from build123d import *

# Parameters (mm, degrees)
BOSS_EXTRUDE1_DEPTH = 6


with BuildPart() as part:
    # Sketch1 → Boss-Extrude1 (new body)
    with BuildSketch(Plane(origin=(0, 0, 0), x_dir=(1, 0, 0), z_dir=(0, 1, 0))):
        with BuildLine():
            ThreePointArc((-521.750777563, 295.459449184), (-519.268832109, 299.8), (-516.750777563, 304.119703222))
            ThreePointArc((-516.750777563, 304.119703222), (-425.745445365, 422.209634839), (-308.418556675, 514.196610158))
            Line((-308.418556675, 514.196610158), (-176.260254038, 285.291715349))
            Line((-176.260254038, 285.291715349), (-171.260254038, 276.631461311))
            Line((-171.260254038, 276.631461311), (-89.706166951, 135.375638912))
            ThreePointArc((-89.706166951, 135.375638912), (-140.642525575, 81.2), (-162.091825827, 10))
            Line((-162.091825827, 10), (-325.2, 10))
            Line((-325.2, 10), (-335.2, 10))
            Line((-335.2, 10), (-599.516605275, 10))
            ThreePointArc((-599.516605275, 10), (-578.516992176, 157.601553812), (-521.750777563, 295.459449184))
        make_face()
    extrude(amount=BOSS_EXTRUDE1_DEPTH)


solid = part.part
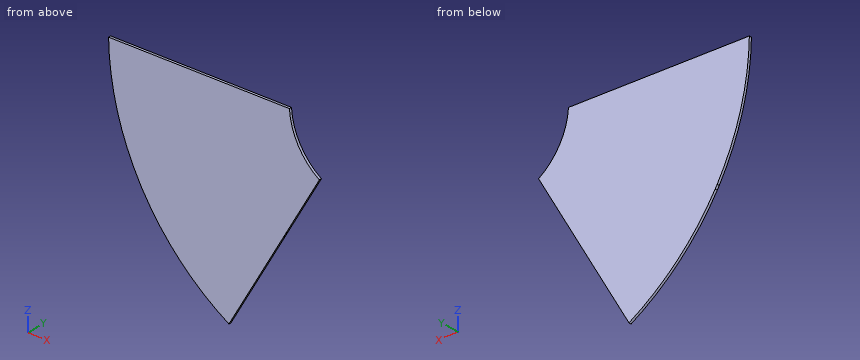
Read the model definition and answer for the solid it produces. Units are mm, in the model's axes. Coordinates: 2 decimals unless noted, no trailing zeros. Order: outer loops, then holes, each group sorted by start corner. A loop starts at its lowest first (then second) coordinate and runs counter-clockwise, first axis right, second up. Notation, with made-up numbers: M 63,5 L 85,5 A22 ccw 85,33 Z; hole C 83.5,-3.75 d7. An arc over 180 degrees is marked long. Put each result on its own line as item: value. Start each with the question number.
Item 1: Section B-B, the plane z = -206.5 is taken. Determine the outline of the cut face in (x, y).
Item 2: Section C-C, the plane x = -456 is taken. Determine the outline of the cut face in (y, z), plus the area to 3 significant figures.
Item 3: Given pin 1 Ø2 at (x, y) = (-461.5, 5) entering from -Z; pin 2 Ø1 at (x, y) = (-231.5, 4.5) entering from -Z; pin 3 Ø1.5 at (y, z) = (3, -440.5) entering from +X, each flat-ended and moving along its own axis, determine where each tip first touches the part or whether it passes through.
Item 4: Consider probe 1 along Z at (x, y) = (-353, 1.25); probe 2 along Z at (x, y) = (-295, 0.6); probe 3 along X at (y, z) = (2.55, -96). Determine where each line is inside the solid, lowest interval first. Write a range as [from, to].
Item 5: Section A-A, the plane y = 4.05 is taken. Determine the outline of the cut face in (x, z).
Computed:
1. outline: M -562.92,0 L -130.77,0 L -130.77,6 L -562.92,6 Z
2. outline: M 0,-389.34 L 6,-389.34 L 6,-10 L 0,-10 Z
2. area: 2,280 mm2
3. pin 1: stops at z = -384.01
3. pin 2: stops at z = -381.84
3. pin 3: stops at x = -265.44
4. probe 1: z = [-484.68, -10]
4. probe 2: z = [-490.95, -10]
4. probe 3: x = [-591.86, -130.99]
5. outline: M -599.52,-10 A599.6 ccw -521.75,-295.46 A599.6 ccw -516.75,-304.12 A599.6 ccw -308.42,-514.2 L -89.71,-135.38 A162.4 cw -162.09,-10 Z
